```python
from build123d import *

# Parameters (mm, degrees)
F0_R     = 1.5
F1_DEPTH = 3


with BuildPart() as f1:
    # F0 (on Front) → F1 (new body)
    with BuildSketch(Plane.XZ):
        with BuildLine():
            ThreePointArc((20.225425, 14.694631), (7.725425, 23.776413), (-7.725425, 23.776413))
            ThreePointArc((-7.725425, 23.776413), (-20.225425, 14.694631), (-25, 0))
            ThreePointArc((-25, 0), (-20.225425, -14.694631), (-7.725425, -23.776413))
            ThreePointArc((-7.725425, -23.776413), (7.725425, -23.776413), (20.225425, -14.694631))
            ThreePointArc((20.225425, -14.694631), (25, 0), (20.225425, 14.694631))
        make_face()
        with Locations((-15.20821, -11.049411)):
            Circle(F0_R, mode=Mode.SUBTRACT)
        with Locations((5.809019, -17.878323)):
            Circle(F0_R, mode=Mode.SUBTRACT)
        with Locations((-15.20821, 11.049411)):
            Circle(F0_R, mode=Mode.SUBTRACT)
        with BuildLine():
            ThreePointArc((-11, 0), (-8.899187, 6.465638), (-3.399187, 10.461622))
            ThreePointArc((-3.399187, 10.461622), (3.399187, 10.461622), (8.899187, 6.465638))
            ThreePointArc((8.899187, 6.465638), (11, 0), (8.899187, -6.465638))
            ThreePointArc((8.899187, -6.465638), (3.399187, -10.461622), (-3.399187, -10.461622))
            ThreePointArc((-3.399187, -10.461622), (-8.899187, -6.465638), (-11, 0))
        make_face(mode=Mode.SUBTRACT)
        with Locations((18.798381, 0)):
            Circle(F0_R, mode=Mode.SUBTRACT)
        with Locations((5.809019, 17.878323)):
            Circle(F0_R, mode=Mode.SUBTRACT)
    extrude(amount=F1_DEPTH)


solid = f1.part
```
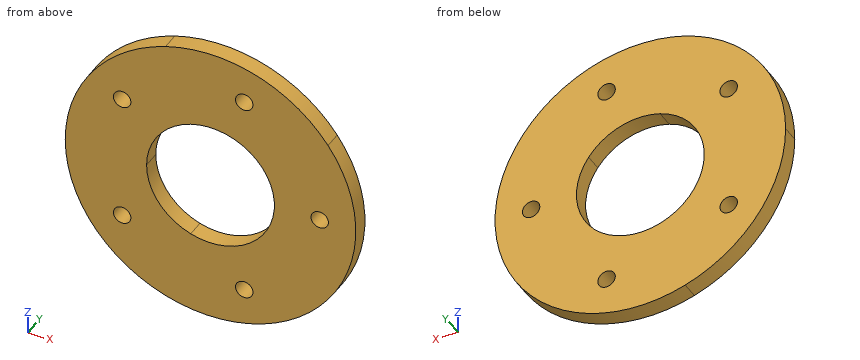
Input: part model. Units: mm. Frame: model coordinates. Give positions to 0.01 mm unless a question says otherwise; leave off trailing zeros. Loops run counter-clockwise (first coordinate to the right, second up) from the corner with the lowest first, then second, coordinate; pieces in that order, holes last. Notation, with made-up numbers: M 22,74 L 32,74 A22 ccw 32,92 Z; hole C -24.5,40.25 d3. An arc over 180 degrees is marked long. Answer as CSV lines item,"result". Start each with the question number.
1. Pin query (flat end, axial travel): P1, Ø1.5, axis at x = -15, y = -1, coming from the -Z side. Return the tip coordinate at first contact, or that it passes through.
2. Section B-B on z = -4. Return loops of the section in (x, y), plus the area to 3 significant figures.
3. Section A-A on x = -1. Return loops of the section in (y, z).
4. Section C-C on y = -1.8. Return loops of the section in (x, z).
5. Section D-D on z = -14. Return loops of the section in (x, y), plus the area to 3 significant figures.
6. Line query: L1, parallel to X at y = -2.15, z = -10; L2, parallel to Z at x = 6.5, y = -2.25; L3, parallel to Z at x = -8.5, y = -0.7. Output: solid intervals per line, ascending.
Computed values:
1,P1,"stops at z = -20.54"
2,outline,"M -24.68,-3 L -10.25,-3 L -10.25,0 L -24.68,0 Z; M 10.25,-3 L 24.68,-3 L 24.68,0 L 10.25,0 Z"
2,area,"86.6 mm²"
3,outline,"M -3,-24.98 L 0,-24.98 L 0,-10.95 L -3,-10.95 Z; M -3,10.95 L 0,10.95 L 0,24.98 L -3,24.98 Z"
4,outline,"M -7.73,-23.78 A25 ccw 20.23,-14.69 A25 ccw -7.73,23.78 A25 ccw Z; hole C -15.21,-11.05 d3; hole C -15.21,11.05 d3; hole C 5.81,-17.88 d3; hole C 5.81,17.88 d3; hole M 8.9,-6.47 A11 ccw 8.9,6.47 A11 ccw long Z; hole C 18.8,0 d3"
5,outline,"M -20.71,-3 L 20.71,-3 L 20.71,0 L -20.71,0 Z"
5,area,"124 mm²"
6,L1,"x = -22.91 to -16.28, -14.14 to -4.58, 4.58 to 22.91"
6,L2,"z = -24.14 to -19.21, -16.55 to -8.87, 8.87 to 16.55, 19.21 to 24.14"
6,L3,"z = -23.51 to -6.98, 6.98 to 23.51"
